For this review, take the finished solid that the model builds, in its own axes (mm). A direction names the side the tool comes from. Give positions to 0.01 mm unless a question says otherwise; leave off trailing zeros. Write each loop counter-clockwise with the first axis right and the second up, starting at its lowest first coordinate (ties: lowest second). Pieces come first, ordered by that corner, then holes.
Q1. Insertion check: P1, Ø1.5, axis at x = 32.5, y = 2, coming from the +Z side; P2, Ø2, axis at x = 34, y = 2, coming from the -Z side. Each pin has a flat end and moves straight along its axis. Give the tip position at first contact, or say it passes through.
Q2. Mouldability with a two-part tool opening along Z and no side actions: class faces 1 (the flat face through (-21, 2, 0)), 2 (the cylindrical face through (-8.1, 1.97, 11.64)), 3 (the cylindrical face through (-19.859, 2.028, -24.797)) as released by +Z, released by -Z, zero draft, split by the parting line, or undercut.
Q3. Machinability: for faces 4 (the flat face through (31, 2, -17.5)), 5 (the flat face through (10, 0, 0)), 6 (the cylindrical face through (8.1, 1.97, 11.64)), which of the approach directions +Z, -Z, +X, -X, +Y, -Y give a long, thin tool a straight path to every point of the face, cutting with its end or side? Answer none if there is none.
Q4. For line 1 (X direction, y = 2, z = -8); line 2 (Z direction, x = -2.5, y = 3.2); line 3 (Z direction, x = 17.5, y = 1.85), list the stretches that pass through material, from the lowest coordinate up.
Q5. We need section C-C (x = 3). Write out the cut boundary in (y, z), then the cut area to 3 significant figures.
Q6. We need section A-A (x = 31). Write out the cut boundary in (y, z).
Q7. We need section D-D (z = 16.5). Write out the cut boundary in (x, y).
Q8. We need section B-B (z = -6.5). Write out the cut boundary in (x, y), then the cut area to 3 significant figures.
```python
from build123d import *

# Parameters (mm, degrees)
SKETCH1_W               = 42
SKETCH1_H               = 52
BOSS_EXTRUDE1_DEPTH     = 4
SKETCH2_R               = 1.65
CUT_EXTRUDE1_DEPTH      = 1
CUT_EXTRUDE1_DEPTH_BACK = 5
SKETCH3_W               = 20
SKETCH3_H               = 35
BOSS_EXTRUDE2_DEPTH     = 4
FILLET1_R               = 4
CUT_EXTRUDE2_DEPTH      = 1
CUT_EXTRUDE2_DEPTH_BACK = 5
SKETCH5_W               = 18
SKETCH5_H               = 25
CUT_EXTRUDE3_DEPTH      = 1
CUT_EXTRUDE3_DEPTH_BACK = 5
FILLET2_R               = 3


with BuildPart() as part:
    # Sketch1 → Boss-Extrude1 (new body)
    with BuildSketch(Plane(origin=(0, 0, 0), x_dir=(1, 0, 0), z_dir=(0, 1, 0))):
        Rectangle(SKETCH1_W, SKETCH1_H)
    extrude(amount=BOSS_EXTRUDE1_DEPTH)

    # Sketch2 → Cut-Extrude1 (cut, two sides)
    with BuildSketch(Plane(origin=(0, 4, 0), x_dir=(1, 0, 0), z_dir=(0, 1, 0))) as cut_extrude1_sk:
        with Locations((-17.975, 22.4375)):
            Circle(SKETCH2_R)
        with Locations((17.975, 22.4375)):
            Circle(SKETCH2_R)
        with Locations((17.975, -22.4375)):
            Circle(SKETCH2_R)
        with Locations((-17.975, -22.4375)):
            Circle(SKETCH2_R)
    extrude(amount=CUT_EXTRUDE1_DEPTH, mode=Mode.SUBTRACT)
    extrude(cut_extrude1_sk.sketch, amount=-CUT_EXTRUDE1_DEPTH_BACK, mode=Mode.SUBTRACT)

    # Sketch3 → Boss-Extrude2 (add)
    with BuildSketch(Plane(origin=(0, 4, 0), x_dir=(1, 0, 0), z_dir=(0, 1, 0))):
        with Locations((31, 0)):
            Rectangle(SKETCH3_W, SKETCH3_H)
    extrude(amount=-BOSS_EXTRUDE2_DEPTH)

    # Fillet1
    fillet1_edges = [part.edges().sort_by_distance(p)[0] for p in [
        (21, 2, 17.5),
        (21, 2, -17.5),
        (41, 2, -17.5),
        (41, 2, 17.5),
        (21, 2, 26),
        (-21, 2, 26),
        (-21, 2, -26),
        (21, 2, -26),
    ]]
    fillet(fillet1_edges, radius=FILLET1_R)

    # Sketch4 → Cut-Extrude2 (cut, two sides)
    with BuildSketch(Plane(origin=(0, 4, 0), x_dir=(1, 0, 0), z_dir=(0, 1, 0))) as cut_extrude2_sk:
        with BuildLine():
            Line((28.85, -9), (28.85, 9))
            ThreePointArc((28.85, 9), (31, 11.15), (33.15, 9))
            Line((33.15, 9), (33.15, -9))
            ThreePointArc((33.15, -9), (31, -11.15), (28.85, -9))
        make_face()
    extrude(amount=CUT_EXTRUDE2_DEPTH, mode=Mode.SUBTRACT)
    extrude(cut_extrude2_sk.sketch, amount=-CUT_EXTRUDE2_DEPTH_BACK, mode=Mode.SUBTRACT)

    # Sketch5 → Cut-Extrude3 (cut, two sides)
    with BuildSketch(Plane(origin=(0, 4, 0), x_dir=(1, 0, 0), z_dir=(0, 1, 0))) as cut_extrude3_sk:
        Rectangle(SKETCH5_W, SKETCH5_H)
    extrude(amount=CUT_EXTRUDE3_DEPTH, mode=Mode.SUBTRACT)
    extrude(cut_extrude3_sk.sketch, amount=-CUT_EXTRUDE3_DEPTH_BACK, mode=Mode.SUBTRACT)

    # Fillet2
    fillet2_edges = [part.edges().sort_by_distance(p)[0] for p in [
        (9, 2, -12.5),
        (9, 2, 12.5),
        (-9, 2, 12.5),
        (-9, 2, -12.5),
    ]]
    fillet(fillet2_edges, radius=FILLET2_R)


solid = part.part
```
Computed:
1. P1: stops at z = 17.5
1. P2: stops at z = -17.5
2. face 1: zero draft
2. face 2: undercut
2. face 3: released by -Z
3. face 4: -Z, +X, +Y, -Y
3. face 5: +Z, -Z, +X, -X, -Y
3. face 6: +Y, -Y
4. line 1: x = -21 to -9, 9 to 28.85, 33.15 to 41
4. line 2: z = -26 to -12.5, 12.5 to 26
4. line 3: z = -25.97 to -24.02, -20.86 to 20.86, 24.02 to 25.97
5. outline: (0, -26) - (4, -26) - (4, -12.5) - (0, -12.5) - close; (0, 12.5) - (4, 12.5) - (4, 26) - (0, 26) - close
5. area: 108 mm2
6. outline: (0, -17.5) - (4, -17.5) - (4, -11.15) - (0, -11.15) - close; (0, 11.15) - (4, 11.15) - (4, 17.5) - (0, 17.5) - close
7. outline: (-21, 0) - (39.65, 0) - (39.65, 4) - (-21, 4) - close
8. outline: (-21, 0) - (-9, 0) - (-9, 4) - (-21, 4) - close; (9, 0) - (28.85, 0) - (28.85, 4) - (9, 4) - close; (33.15, 0) - (41, 0) - (41, 4) - (33.15, 4) - close
8. area: 159 mm2
